Can you work these out from the model? Positions are in its coordinate system, mm. A direction names the side the tool comes from. Coordinates: 2 decimals unless noted, no trailing zeros. Order: outer loops, then holes, each group sorted by start corner. A loop starts at its lowest first (then second) coordinate and runs counter-clockwise, first axis right, second up. Notation, with made-up numbers: (-35.75, 10.25) -> (7.25, 10.25) arc R19 ccw to (7.25, 14.25) -> close; hole circle Ø11 at (-12.5, -4.75). An arc over 180 degrees is marked (long way). Answer in a Markdown table with one row per item.
```python
from build123d import *

# Parameters (mm, degrees)
SKETCH1_R           = 5
BOSS_EXTRUDE1_DEPTH = 130
CUT_EXTRUDE1_DEPTH  = 131.479883507
SKETCH3_R           = 2
CUT_EXTRUDE2_DEPTH  = 131.479883618
CHAMFER1_SIZE       = 0.5


with BuildPart() as part:
    # Sketch1 → Boss-Extrude1 (new body)
    with BuildSketch(Plane.XY):
        Circle(SKETCH1_R)
    extrude(amount=BOSS_EXTRUDE1_DEPTH)

    # Sketch2 → Cut-Extrude1 (cut, through all)
    with BuildSketch(Plane(origin=(0, 5, 0), x_dir=(1, 0, 0), z_dir=(0, 1, 0))):
        with BuildLine():
            Line((-3, 0), (3, 0))
            Line((3, 0), (3, -8))
            ThreePointArc((3, -8), (0, -11), (-3, -8))
            Line((-3, -8), (-3, 0))
        make_face()
    extrude(amount=-CUT_EXTRUDE1_DEPTH, mode=Mode.SUBTRACT)

    # Sketch3 → Cut-Extrude2 (cut, through all)
    with BuildSketch(Plane(origin=(5, 0, 0), x_dir=(0, 0, -1), z_dir=(1, 0, 0))):
        with Locations((-4, 0)):
            Circle(SKETCH3_R)
        Polygon((-8, -4), (0, -1), (0, -4), align=None)
        Polygon((0, 1), (0, 4), (-8, 4), align=None)
    extrude(amount=-CUT_EXTRUDE2_DEPTH, mode=Mode.SUBTRACT)

    # Chamfer1
    chamfer1_edges = [part.edges().sort_by_distance(p)[0] for p in [
        (-3.949489743, -1, 0),
        (-5, 0, 0),
        (4.974680765, -0.50254481, 0),
        (-3.949489743, 1, 0),
        (-3, 0, 0),
        (3, 0, 0),
        (3.949489743, -1, 0),
        (3.949489743, 1, 0),
    ]]
    chamfer(chamfer1_edges, length=CHAMFER1_SIZE)


solid = part.part
```
(1) On a 3-axis mill with a long thin cutter (end or side, diameter ignored), from which of +Z, -Z, +X, -X, +Y, -Y can I reach the whole of each face in a straight line? I mean faces 5 (the cylindrical face through (-5, 0, 64)), 6 (the flat face through (-3, -1, 6)). Say none if no direction works.
Response values:
| item | result |
|---|---|
| face 5 | +Z, -Z |
| face 6 | -Z, +Y, -Y |
(2) We'd pull the mould along Y, two halves only. Please class faces 1 (the flat face through (3.735, 2.294, 3.45)), 2 (the flat face through (-3.709, -2.294, 3.45)), 3 (the flat face through (0, 0, 130)), 4 (the cylindrical face through (4.014, 1.686, 2.925)): +Y half, -Y half, draft (parallel to the pull), parting line (faces both ways), or undercut.
Response values:
| item | result |
|---|---|
| face 1 | +Y half |
| face 2 | -Y half |
| face 3 | draft |
| face 4 | undercut |
(3) Suppose I cut it at C-C (x = -1.75). Please give me the cut outline in (y, z).
Response values:
| item | result |
|---|---|
| outline | (-4.68, 10.44) -> (4.68, 10.44) -> (4.68, 130) -> (-4.68, 130) -> close |
(4) I need wall thicknesses on line 1 (Z direction, x = -3.7, y = 0); line 2 (X direction, y = -4, z = 86.5); line 3 (Z direction, x = 0, y = 2). Which ranges of each line are inside material? Lowest first, please. Write a range as [from, to].
Response values:
| item | result |
|---|---|
| line 1 | [0, 2], [6, 130] |
| line 2 | [-3, 3] |
| line 3 | [11, 130] |
(5) Suppose I cut it at B-B (z = 19). Please give me the cut outline in (x, y), and give its area (3 significant figures).
Response values:
| item | result |
|---|---|
| outline | circle Ø10 at (0, 0) |
| area | 78.5 mm2 |
(6) Suppose I cut it at A-A (z = 4). Please give me the cut outline in (x, y), and give its area (3 significant figures).
Response values:
| item | result |
|---|---|
| outline | (-4.58, -2) arc R5 ccw to (-4.33, -2.5) -> (-3, -2.5) -> (-3, -2) -> close; (-4.58, 2) -> (-3, 2) -> (-3, 2.5) -> (-4.33, 2.5) arc R5 ccw to start; (3, -2.5) -> (4.33, -2.5) arc R5 ccw to (4.58, -2) -> (3, -2) -> close; (3, 2) -> (4.58, 2) arc R5 ccw to (4.33, 2.5) -> (3, 2.5) -> close |
| area | 2.92 mm2 |
(7) Will this pin go through, and if not, where does the flat tip stop? pin 1 Ø3 at (y, z) = (-1, 81) entering from +X.
Response values:
| item | result |
|---|---|
| pin 1 | x = 5 |
